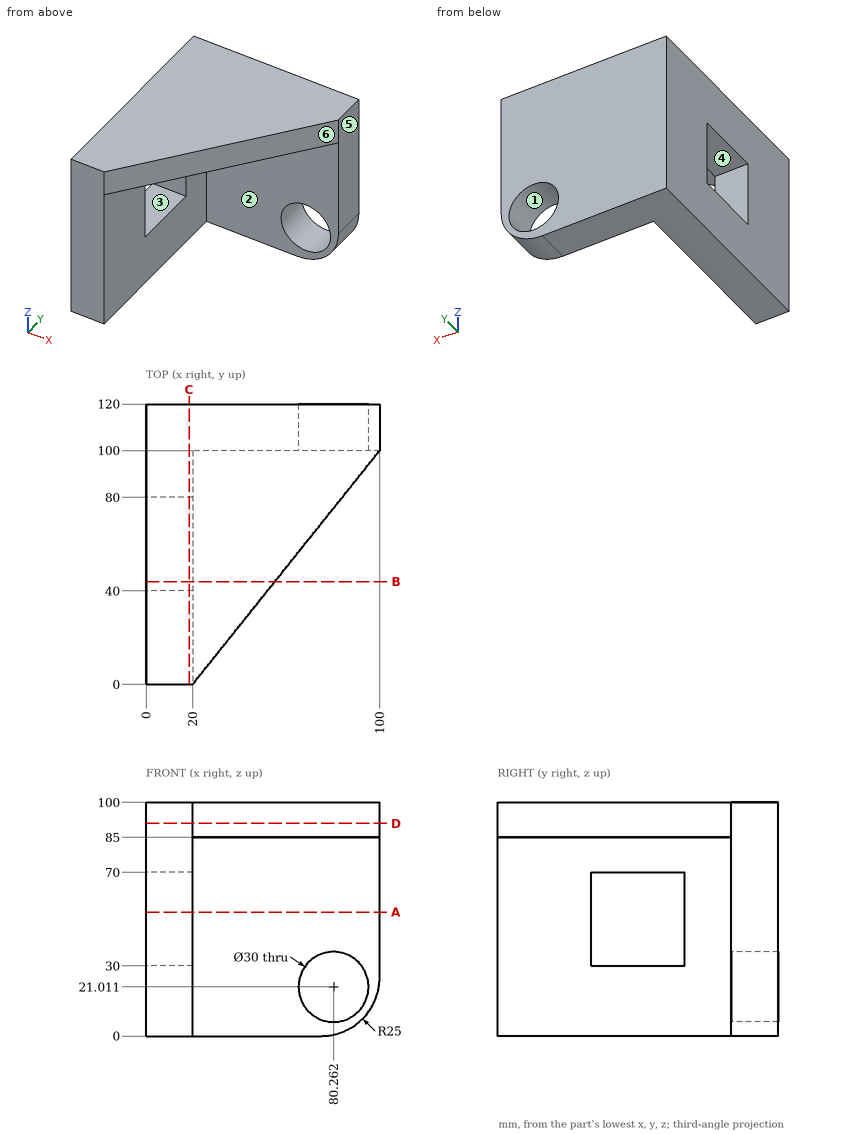
For this review, use the dimensioned drawing (mm, ordinates from the lowest corner) and the shaded views. A direction names the side the tool comes from. Coordinates: 2 decimals unless noted, no trailing zeros. Loops run counter-clockwise (first coordinate to the right, second up) from the corner with the lowest first, then second, coordinate; pieces in that order, holes last. Notation, with made-up numbers: (3, 10) -> (50, 10) arc R21 ccw to (50, 32) -> close; hole circle Ø6 at (33, 86). An arc over 180 degrees is marked (long way). Use a Markdown table: item, result. Add a question column.
Item 1: Clearance check with flat-ended pins moving along their axes: P1, Ø2, axis at x = 23.5, y = 89.5, coming from the -Z side; P2, Ø8, axis at y = 40, z = 26, coming from the +X side. State where each tip first meets the part, or that it passes through.
Item 2: We need section A-A, the plane z = 53. Write out the cut boundary in (x, y), and give its area (3 significant figures).
Item 3: Machinability: for the marked faces 1, 2 and 3, which of the approach directions +Z, -Z, +X, -X, +Y, -Y give a long, thin tool a straight path to every point of the face, cutting with its end or side? Answer none if there is none.
Item 4: The part is to be moulded in two halves that separate along Y. For the marked faces 4, 5 and 6, say which applies: +Y half, -Y half, draft (parallel to the pull), parting line (faces both ways), or undercut.
Item 5: We need section B-B, the plane y = 44. Write out the cut boundary in (x, z).
Item 6: Wall thickness on L1, parallel to Z at x = 18, y = 51; L2, parallel to X at y = 5.5, z = 74; L3, parallel to Z at x = 37, y = 46: over which ranges is each line inside the solid? List them lowest first. Write a range as from..to.
Item 7: We need section C-C, the plane x = 18.5. Write out the cut boundary in (y, z), and give its area (3 significant figures).
Item 8: We need section D-D, the plane z = 91. Write out the cut boundary in (x, y), and give its area (3 significant figures).
Numbers:
| question | item | result |
|---|---|---|
| 1 | P1 | stops at z = 85 |
| 1 | P2 | stops at x = 20 |
| 2 | outline | (0, 0) -> (20, 0) -> (20, 40) -> (0, 40) -> close; (0, 80) -> (20, 80) -> (20, 100) -> (100, 100) -> (100, 120) -> (0, 120) -> close |
| 2 | area | 3,200 mm^2 |
| 3 | face 1 | +Y, -Y |
| 3 | face 2 | -Z, +X, -Y |
| 3 | face 3 | +X, -X |
| 4 | face 4 | undercut |
| 4 | face 5 | draft |
| 4 | face 6 | -Y half |
| 5 | outline | (0, 0) -> (20, 0) -> (20, 30) -> (0, 30) -> close; (0, 70) -> (20, 70) -> (20, 85) -> (55.2, 85) -> (55.2, 100) -> (0, 100) -> close |
| 6 | L1 | z = 0..30, 70..100 |
| 6 | L2 | x = 0..20 |
| 6 | L3 | z = 85..100 |
| 7 | outline | (0, 0) -> (120, 0) -> (120, 100) -> (0, 100) -> close; hole (40, 30) -> (80, 30) -> (80, 70) -> (40, 70) -> close |
| 7 | area | 10,400 mm^2 |
| 8 | outline | (0, 0) -> (20, 0) -> (100, 100) -> (100, 120) -> (0, 120) -> close |
| 8 | area | 8,000 mm^2 |
